Build history of the part. All positions in model axes, mm. A direction names the side the tool comes from. Give positions to 0.01 mm unless a question says otherwise; leave off trailing zeros. Order: outer loops, then holes, each group sorted by start corner. A loop starts at its lowest first (then second) coordinate and runs counter-clockwise, first axis right, second up. Notation, with made-up numbers: M 48,57.5 L 91,57.5 A22 ccw 91,93.5 Z; hole C 30,72 d8. An arc over 180 degrees is marked long. One line per item, written item: value.
from build123d import *

# Parameters (mm, degrees)
SKETCH1_R           = 32.5
BOSS_EXTRUDE1_DEPTH = 12.5
SKETCH2_R           = 32.5
BOSS_EXTRUDE2_DEPTH = 80
SKETCH3_R           = 32.5
BOSS_EXTRUDE3_DEPTH = 12.5


with BuildPart() as part:
    # Sketch1 → Boss-Extrude1 (new body)
    with BuildSketch(Plane(origin=(0, 0, 0), x_dir=(0, 0, -1), z_dir=(1, 0, 0))):
        with BuildLine():
            Line((-52, 48), (-52, -48))
            Line((-52, -48), (0, -48))
            ThreePointArc((0, -48), (48, 0), (0, 48))
            Line((0, 48), (-52, 48))
        make_face()
        Circle(SKETCH1_R, mode=Mode.SUBTRACT)
    extrude(amount=BOSS_EXTRUDE1_DEPTH)

    # Sketch2 → Boss-Extrude2 (add)
    with BuildSketch(Plane(origin=(12.5, 0, 0), x_dir=(0, 0, -1), z_dir=(1, 0, 0))):
        with BuildLine():
            Line((0, 40), (-44, 40))
            Line((-44, 40), (-44, -40))
            Line((-44, -40), (0, -40))
            ThreePointArc((0, -40), (40, 0), (0, 40))
        make_face()
        Circle(SKETCH2_R, mode=Mode.SUBTRACT)
    extrude(amount=BOSS_EXTRUDE2_DEPTH)

    # Sketch3 → Boss-Extrude3 (add)
    with BuildSketch(Plane(origin=(92.5, 0, 0), x_dir=(0, 0, -1), z_dir=(1, 0, 0))):
        with BuildLine():
            Line((0, 48), (-52, 48))
            Line((-52, 48), (-52, -48))
            Line((-52, -48), (0, -48))
            ThreePointArc((0, -48), (48, 0), (0, 48))
        make_face()
        Circle(SKETCH3_R, mode=Mode.SUBTRACT)
    extrude(amount=BOSS_EXTRUDE3_DEPTH)


solid = part.part
1) Saw through at B-B, the plane y = -7. Write the cut outline in (x, z).
Check values:
outline: M 0,-47.49 L 12.5,-47.49 L 12.5,-39.38 L 92.5,-39.38 L 92.5,-47.49 L 105,-47.49 L 105,-31.74 L 0,-31.74 Z; M 0,31.74 L 105,31.74 L 105,52 L 92.5,52 L 92.5,44 L 12.5,44 L 12.5,52 L 0,52 Z
2) Drill centre lines: probe 1 along Y at (x, z) = (32, 0); probe 2 along X at (y, z) = (-29, 45.5); probe 3 along Z at (x, y) = (43, 7). Where is each one in solid material? Low to high. Write a range as from..to.
Check values:
probe 1: -40..-32.5, 32.5..40
probe 2: 0..12.5, 92.5..105
probe 3: -39.38..-31.74, 31.74..44
3) Mould opens along X. For faces 5 (the face through (6, 1, 52)), 6 (the face through (105, 22, 25)), 7 (the face through (51.94, -0.88, -39.99)), 8 (the face through (0, 22, 25)) say: released by +X, released by -X, zero draft, split by the parting line, or undercut.
Check values:
face 5: zero draft
face 6: released by +X
face 7: undercut
face 8: released by -X
4) Saw through at C-C, the plane x = 62. Write the cut outline in (y, z).
Check values:
outline: M -40,0 A40 ccw 40,0 L 40,44 L -40,44 Z; hole C 0,0 d65
5) Tool access for faces 1 (the face through (52, -40, 22)), 2 (the face through (52, 40, 22)), 3 (the face through (12.5, 4, 47)), 4 (the face through (52, 1, 44)): list every direction of +Z, -Z, +X, -X, +Y, -Y with a clear straight run to the whole face (end or side of a thin tool).
Check values:
face 1: +Z, -Z, -Y
face 2: +Z, -Z, +Y
face 3: none
face 4: +Z, +Y, -Y
6) Saw through at A-A, the plane z = -41.5. Write the cut outline in (x, y), then the cut area to 3 significant figures.
Check values:
outline: M 0,-24.12 L 12.5,-24.12 L 12.5,24.12 L 0,24.12 Z; M 92.5,-24.12 L 105,-24.12 L 105,24.12 L 92.5,24.12 Z
area: 1,210 mm^2
7) Saw through at D-D, the plane z = -8.5. Write the cut outline in (x, y), then the cut area to 3 significant figures.
Check values:
outline: M 0,-47.24 L 12.5,-47.24 L 12.5,-39.09 L 92.5,-39.09 L 92.5,-47.24 L 105,-47.24 L 105,-31.37 L 0,-31.37 Z; M 0,31.37 L 105,31.37 L 105,47.24 L 92.5,47.24 L 92.5,39.09 L 12.5,39.09 L 12.5,47.24 L 0,47.24 Z
area: 2,030 mm^2
8) Pin check, flat tips, straight feed: pin 1 (10 mm diameter, centred on x = 12.5, y = -24.5, fed in from -Z); pin 2 (2 mm diameter, centred on x = 24.5, z = 17, fed in from +Y); pin 3 (22 mm diameter, centred on x = 33, z = 12.5, fed in from -Y). Stop position of each tip, or through.
Check values:
pin 1: z = -43.86
pin 2: y = 40
pin 3: y = -40
